```python
from build123d import *

# Parameters (mm, degrees)
F1_DEPTH = 1
F3_D     = 3.6
F4_SIZE  = 5


with BuildPart() as f1:
    # F0 (on Top) → F1 (new body)
    with BuildSketch(Plane.XY):
        with BuildLine():
            Line((41.9170247219, -17.6387755275), (41.9170247219, 16.3612244725))
            Line((41.9170247219, 16.3612244725), (-38.0829752781, 16.3612244725))
            ThreePointArc((-38.0829752781, 16.3612244725), (-41.618509184, 14.8967583785), (-43.0829752781, 11.3612244725))
            Line((-43.0829752781, 11.3612244725), (-43.0829752781, -12.6387755275))
            ThreePointArc((-43.0829752781, -12.6387755275), (-41.618509184, -16.1743094334), (-38.0829752781, -17.6387755275))
            Line((-38.0829752781, -17.6387755275), (41.9170247219, -17.6387755275))
        make_face()
    extrude(amount=F1_DEPTH)

    # F3 (through all)
    with Locations(Plane(origin=(0, 0, 0), x_dir=(1, 0, 0), z_dir=(0, 0, -1))):
        with Locations((-25.6229752781, 13.9887755275), (14.3770247219, -6.0112244725)):
            Hole(F3_D / 2)

    # F4
    f4_edges = [f1.edges().sort_by_distance(p)[0] for p in [
        (41.917025, -17.638776, 0.5),
    ]]
    chamfer(f4_edges, length=F4_SIZE)


solid = f1.part
```
Geometry: final body of the model. Coordinates: model frame, mm. Round coordinates to 2 decimals unless told otherwise and drop trailing zeros. Order: outer loops, then holes, each group sorted by start corner. A loop starts at its lowest first (then second) coordinate and runs counter-clockwise, first axis right, second up. Notation, with made-up numbers: (-1, 60.25) -> (44, 60.25) arc R28 cw to (44, 95.25) -> close; hole circle Ø2 at (-23.75, 63.5). An arc over 180 degrees is marked (long way). Use one line per item in the form item = value. Start each with the question number.
1. Pin query (flat end, axial travel): pin 1 Ø3 at (x, y) = (-25.62, -13.99) entering from +Z. Return the tip coordinate at first contact, or that it passes through.
2. Cut plane A-A (z = 0.15). Return the cut outline in (x, y).
3. Line query: probe 1 along X at (y, z) = (6.5, 0.55); probe 2 along X at (y, z) = (7.5, 0.8); probe 3 along Y at (x, z) = (-25, 0.15). Output: solid intervals per line, ascending.
4. Draft query along X for faces 1 (the face through (-1, 0, 1)), 2 (the face through (16.175, 5.932, 0.507)), 3 (the face through (-26.45, -12.39, 0.51)), 4 (the face through (39.382, -15.174, 0.493)). Return one class per face: pulls with the +X half, pulls with the -X half, needs draft (parallel to the pull), parting line crosses it, or undercut.
Solution:
q1.pin_1 = through
q2.outline = (-43.08, -12.64) arc R5 ccw to (-38.08, -17.64) -> (36.92, -17.64) -> (41.92, -12.64) -> (41.92, 16.36) -> (-38.08, 16.36) arc R5 ccw to (-43.08, 11.36) -> close; hole circle Ø3.6 at (-25.62, -13.99); hole circle Ø3.6 at (14.38, 6.01)
q3.probe_1 = -43.08 to 12.64, 16.11 to 41.92
q3.probe_2 = -43.08 to 13.37, 15.39 to 41.92
q3.probe_3 = -17.64 to -15.68, -12.3 to 16.36
q4.face_1 = needs draft
q4.face_2 = undercut
q4.face_3 = undercut
q4.face_4 = pulls with the +X half
